Check sheet for the modelled part. Datum: model origin and axes. Units: mm. Give positions to 0.01 mm unless a question says otherwise; leave off trailing zeros. Write each loop counter-clockwise with the first axis right and the second up, starting at its lowest first coordinate (ties: lowest second). Pieces come first, ordered by that corner, then holes. Notation, with made-up numbers: M 71,-32 L 107,-32 A20 ccw 107,1 Z; hole C 10.5,84.25 d1. An arc over 180 degrees is marked long. One line per item, written item: value. Start each with the question number.
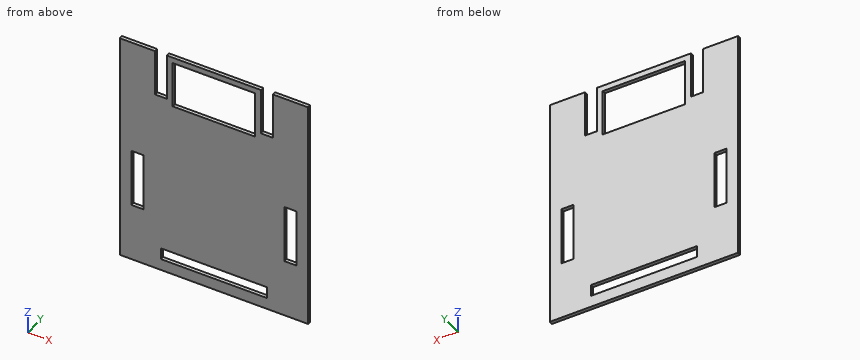
from build123d import *

# Parameters (mm, degrees)
SKETCH1_W           = 10
SKETCH1_H           = 50
BOSS_EXTRUDE1_DEPTH = 3


with BuildPart() as part:
    # Sketch1 → Boss-Extrude1 (new body)
    # profile 1 of 2: a face of its own
    with BuildSketch(Plane(origin=(0, 0, 0), x_dir=(1, 0, 0), z_dir=(0, 1, 0))):
        Polygon((50.939044481, 91.268533773), (-29.060955519, 91.268533773), (-29.060955519, 81.268533773), (15.939044481, 81.268533773), (15.939044481, 71.268533773), (-29.060955519, 71.268533773), (-29.060955519, -63.731466227), (5.939044481, -63.731466227), (5.939044481, -103.731466227), (-29.060955519, -103.731466227), (-29.060955519, -108.731466227), (10.939044481, -108.731466227), (10.939044481, -68.731466227), (20.939044481, -68.731466227), (20.939044481, -108.731466227), (50.939044481, -108.731466227), align=None)
        with Locations((35.939044481, 16.268533773)):
            Rectangle(SKETCH1_W, SKETCH1_H, mode=Mode.SUBTRACT)
    # profile 2 of 2: a face of its own
    with BuildSketch(Plane(origin=(0, 0, 0), x_dir=(1, 0, 0), z_dir=(0, 1, 0))):
        Polygon((-29.060955519, 81.268533773), (-29.060955519, 91.268533773), (-109.060955519, 91.268533773), (-109.060955519, -108.731466227), (-79.060955519, -108.731466227), (-79.060955519, -68.731466227), (-69.060955519, -68.731466227), (-69.060955519, -108.731466227), (-29.060955519, -108.731466227), (-29.060955519, -103.731466227), (-64.060955519, -103.731466227), (-64.060955519, -63.731466227), (-29.060955519, -63.731466227), (-29.060955519, 71.268533773), (-74.060955519, 71.268533773), (-74.060955519, 81.268533773), align=None)
        with Locations((-94.060955519, 16.268533773)):
            Rectangle(SKETCH1_W, SKETCH1_H, mode=Mode.SUBTRACT)
    extrude(amount=BOSS_EXTRUDE1_DEPTH)


solid = part.part
1) Cross-section at C-C (z = 0). Record the boundary of the cut face in (x, y).
2) Cross-section at B-B (x = -16.5). Record the boundary of the cut face in (y, z).
3) Cross-section at A-A (z = 89.5). Record the boundary of the cut face in (x, y), plus the area to 3 significant figures.
4) Material ranges on L1, parallel to Z at x = -51.5, y = 1.4; L2, parallel to X at y = 1.75, z = 4; L3, parallel to X at y = 1.15, z = -77.5, recorded low to high. Write a range as from..to.
5) Cross-section at D-D (x = 13). Record the boundary of the cut face in (y, z), plus the area to 3 significant figures.
Data:
1. outline: M -109.06,0 L -99.06,0 L -99.06,3 L -109.06,3 Z; M -89.06,0 L 30.94,0 L 30.94,3 L -89.06,3 Z; M 40.94,0 L 50.94,0 L 50.94,3 L 40.94,3 Z
2. outline: M 0,-91.27 L 3,-91.27 L 3,-81.27 L 0,-81.27 Z; M 0,-71.27 L 3,-71.27 L 3,63.73 L 0,63.73 Z; M 0,103.73 L 3,103.73 L 3,108.73 L 0,108.73 Z
3. outline: M -109.06,0 L -79.06,0 L -79.06,3 L -109.06,3 Z; M -69.06,0 L -64.06,0 L -64.06,3 L -69.06,3 Z; M 5.94,0 L 10.94,0 L 10.94,3 L 5.94,3 Z; M 20.94,0 L 50.94,0 L 50.94,3 L 20.94,3 Z
3. area: 210 mm2
4. L1: z = -91.27..-81.27, -71.27..63.73, 103.73..108.73
4. L2: x = -109.06..-99.06, -89.06..30.94, 40.94..50.94
4. L3: x = -109.06..-74.06, 15.94..50.94
5. outline: M 0,-91.27 L 3,-91.27 L 3,-81.27 L 0,-81.27 Z; M 0,-71.27 L 3,-71.27 L 3,68.73 L 0,68.73 Z
5. area: 450 mm2
